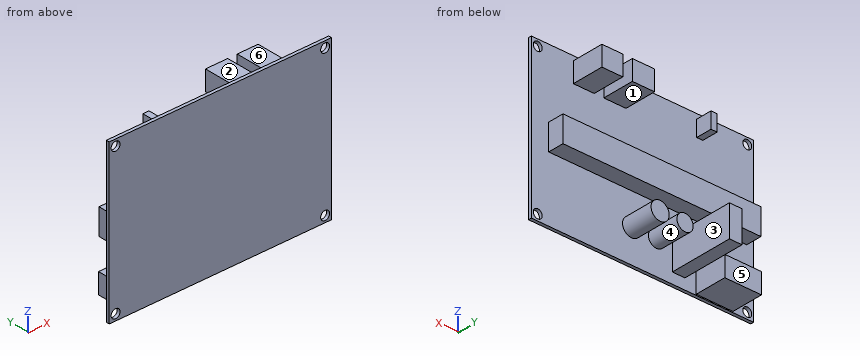
from build123d import *

# Parameters (mm, degrees)
SKETCH1_W           = 70
SKETCH1_H           = 50
BOSS_EXTRUDE1_DEPTH = 1
SKETCH2_R           = 1.4
CUT_EXTRUDE1_DEPTH  = 87.029064856
SKETCH3_R           = 2.564653552
SKETCH3_R_2         = 2.860541453
SKETCH3_W           = 6.997065393
SKETCH3_H           = 6.279852664
SKETCH3_W_2         = 6.578665668
SKETCH3_W_3         = 11.565083488
SKETCH3_H_2         = 6.404713395
BOSS_EXTRUDE2_DEPTH = 10
SKETCH5_W           = 62.355948398
SKETCH5_H           = 8.179994237
SKETCH5_W_2         = 1.926807787
SKETCH5_H_2         = 5.042884886
BOSS_EXTRUDE3_DEPTH = 5
SKETCH6_W           = 3.975602045
SKETCH6_H           = 9.897897773
BOSS_EXTRUDE4_DEPTH = 20


with BuildPart() as part:
    # Sketch1 → Boss-Extrude1 (new body)
    with BuildSketch(Plane(origin=(0, 0, 0), x_dir=(1, 0, 0), z_dir=(0, 1, 0))):
        with Locations((35, 25)):
            Rectangle(SKETCH1_W, SKETCH1_H)
    extrude(amount=BOSS_EXTRUDE1_DEPTH)

    # Sketch2 → Cut-Extrude1 (cut, through all)
    with BuildSketch(Plane(origin=(0, 1, 0), x_dir=(1, 0, 0), z_dir=(0, 1, 0))):
        with Locations(Location((2, 48, 0), (0, 0, 270))):
            Circle(SKETCH2_R)
        with Locations(Location((68, 48, 0), (0, 0, 270))):
            Circle(SKETCH2_R)
        with Locations(Location((68, 2, 0), (0, 0, 270))):
            Circle(SKETCH2_R)
        with Locations(Location((2, 2, 0), (0, 0, 270))):
            Circle(SKETCH2_R)
    extrude(amount=-CUT_EXTRUDE1_DEPTH, mode=Mode.SUBTRACT)

    # Sketch3 → Boss-Extrude2 (add)
    with BuildSketch(Plane(origin=(0, 1, 0), x_dir=(1, 0, 0), z_dir=(0, 1, 0))):
        with Locations(Location((30.577880589, 39.645889027, 0), (0, 0, 90))):
            Circle(SKETCH3_R)
        with Locations(Location((38.435044471, 39.645889027, 0), (0, 0, 90))):
            Circle(SKETCH3_R_2)
        with Locations((43.70288795, 4.543658094)):
            Rectangle(SKETCH3_W, SKETCH3_H)
        with Locations((53.497105797, 4.543658094)):
            Rectangle(SKETCH3_W_2, SKETCH3_H)
        with Locations((12.304871688, 46.48029873)):
            Rectangle(SKETCH3_W_3, SKETCH3_H_2)
    extrude(amount=BOSS_EXTRUDE2_DEPTH)

    # Sketch5 → Boss-Extrude3 (add)
    with BuildSketch(Plane(origin=(0, 1, 0), x_dir=(1, 0, 0), z_dir=(0, 1, 0))):
        with Locations((33.371807315, 25.517900554)):
            Rectangle(SKETCH5_W, SKETCH5_H)
        with Locations((16.963761322, 4.054342187)):
            Rectangle(SKETCH5_W_2, SKETCH5_H_2)
    extrude(amount=BOSS_EXTRUDE3_DEPTH)

    # Sketch6 → Boss-Extrude4 (add)
    with BuildSketch(Plane(origin=(0, 1, 0), x_dir=(1, 0, 0), z_dir=(0, 1, 0))):
        with Locations((23.62978258, 41.700410586)):
            Rectangle(SKETCH6_W, SKETCH6_H)
    extrude(amount=BOSS_EXTRUDE4_DEPTH)


solid = part.part
Model file for the job. Use its own axes, mm. Face numbers are marked on the shaded views. A direction names the side the tool comes from. Give positions to 0.01 mm unless a question says otherwise; leave off trailing zeros. Order: outer loops, then holes, each group sorted by start corner. A loop starts at its lowest first (then second) coordinate and runs counter-clockwise, first axis right, second up. Notation, with made-up numbers: M -40,7 L 11,7 A24 ccw 11,19 Z; hole C -1,-34.75 d8. An arc over 180 degrees is marked long. Write item = value, one per line.
Q1. Tool access for the marked faces 1, 2 and 3: list every direction of +Z, -Z, +X, -X, +Y, -Y with a clear straight run to the whole face (end or side of a thin tool).
Derived:
face_1 = +X, -X, +Y
face_2 = +Z, +X, -X, +Y
face_3 = -Z, +Y
Q2. Two-plate mould, pull along Z, no slides. Class the marked faces 4, 5 and 6: pulls with the +Z half, pulls with the -Z half, needs draft (parallel to the pull), parting line crosses it, or undercut.
Derived:
face_4 = undercut
face_5 = needs draft
face_6 = pulls with the +Z half
Q3. Drill centre lines: line 1 (Z direction, x = 68, y = 0.55); line 2 (X direction, y = 0.75, z = -48); line 3 (Z direction, x = 45.5, y = 4.75). Where is each one in solid material? Low to high. Write a range as [from, to].
Derived:
line_1 = [-50, -49.4], [-46.6, -3.4], [-0.6, 0]
line_2 = [0, 0.6], [3.4, 66.6], [69.4, 70]
line_3 = [-29.61, -21.43], [-7.68, -1.4]
Q4. Cut at C-C, the plane y = 8.25. List the corners of the cut face in (x, z), then the cut area to 3 significant figures.
Derived:
outline = M 6.52,-49.68 L 18.09,-49.68 L 18.09,-43.28 L 6.52,-43.28 Z; M 21.64,-46.65 L 25.62,-46.65 L 25.62,-36.75 L 21.64,-36.75 Z; C 30.58,-39.65 d5.13; C 38.44,-39.65 d5.72; M 40.2,-7.68 L 47.2,-7.68 L 47.2,-1.4 L 40.2,-1.4 Z; M 50.21,-7.68 L 56.79,-7.68 L 56.79,-1.4 L 50.21,-1.4 Z
area = 245 mm2
Q5. Cut at B-B, the plane z = -48. List the corners of the cut face in (x, y).
Derived:
outline = M 0,0 L 0.6,0 L 0.6,1 L 0,1 Z; M 3.4,0 L 66.6,0 L 66.6,1 L 18.09,1 L 18.09,11 L 6.52,11 L 6.52,1 L 3.4,1 Z; M 69.4,0 L 70,0 L 70,1 L 69.4,1 Z
Q6. Cut at A-A, the plane x = 68. List the corners of the cut face in (y, z), then the cut area to 3 significant figures.
Derived:
outline = M 0,-50 L 1,-50 L 1,-49.4 L 0,-49.4 Z; M 0,-46.6 L 1,-46.6 L 1,-3.4 L 0,-3.4 Z; M 0,-0.6 L 1,-0.6 L 1,0 L 0,0 Z
area = 44.4 mm2
Q7. Cut at D-D, the plane x = 43.5. List the corners of the cut face in (y, z).
Derived:
outline = M 0,-50 L 1,-50 L 1,-29.61 L 6,-29.61 L 6,-21.43 L 1,-21.43 L 1,-7.68 L 11,-7.68 L 11,-1.4 L 1,-1.4 L 1,0 L 0,0 Z
Q8. Flat gauge pins, fed straight in: pin 1 (1.9 mm diameter, centred on y = 6.5, z = -48, fed in from -X); pin 2 (6 mm diameter, centred on x = 43, z = -29, fed in from +Y); pin 3 (8 mm diameter, centred on x = 44.5, y = 14, fed in from -Z). Where does each tip first touch, or does it go through?
Derived:
pin_1 = 6.52
pin_2 = 6
pin_3 = -7.68
